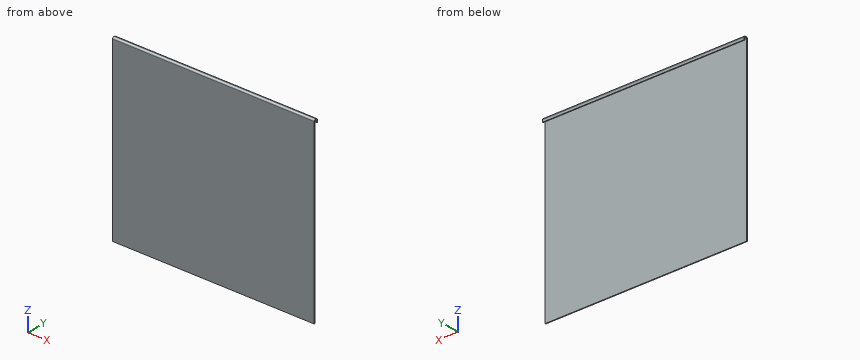
Autodesk Inventor part; units mm, degrees
ref_plane "YZ Plane" through (0, 0, 0) normal (1, 0, 0) x (0, 1, 0)
ref_plane "XZ Plane" through (0, 0, 0) normal (0, 1, 0) x (-1, 0, 0)
ref_plane "XY Plane" through (0, 0, 0) normal (0, 0, 1) x (1, 0, 0)
sketch "Sketch1" plane through (0, 0, 0) normal (0, 1, 0) x (-1, 0, 0)
  line L0 (0, 0) -> (1371.6, 0)
  line L1 (1371.6, 0) -> (1371.6, 1219.2)
  line L2 (1371.6, 1219.2) -> (0, 1219.2)
  line L3 (0, 1219.2) -> (0, 0)
  dimension "d0" = 1371.6
  dimension "d1" = 1219.2
extrude "Plate1" add sketch "Sketch1" along normal blind 5.3975
sketch "Sketch2" plane through (0, 0, 1213.8025) normal (0, 0, 1) x (1, 0, 0)
  line L0 (-1371.6, 0) -> (0, 0)
  line L1 (0, 0) -> (0, 25.4)
  line L2 (0, 25.4) -> (-1371.6, 25.4)
  line L3 (-1371.6, 25.4) -> (-1371.6, 0)
edge flange "Flange1" height 25.4 angle 90 thickness 5.3975 bend radius 5.3975 thickness toward (0, 0, 1) relief tear relief width 5.3975 relief depth 2.6987 edges at (-685.8, 5.3975, 1219.2) wall of the first edge with corners at (-1371.6, 0, 1213.8025) (0, 0, 1213.8025) (0, 25.4, 1213.8025) (-1371.6, 25.4, 1213.8025)
bend "Bend1"
corner "Corner1"
sketch "Sketch3" plane through (0, 20.0025, 1219.2) normal (0, 1, 0) x (-1, 0, 0)
  line L0 (1371.6, 0) -> (0, 0)
  line L1 (0, 0) -> (0, -25.4)
  line L2 (0, -25.4) -> (1371.6, -25.4)
  line L3 (1371.6, -25.4) -> (1371.6, 0)
edge flange "Flange2" height 25.4 angle 90 thickness 5.3975 bend radius 5.3975 thickness toward (0, 1, 0) relief tear relief width 5.3975 relief depth 2.6987 edges at (-685.8, 25.4, 1213.8025) wall of the first edge with corners at (-1371.6, 20.0025, 1219.2) (0, 20.0025, 1219.2) (0, 20.0025, 1193.8) (-1371.6, 20.0025, 1193.8)
bend "Bend2"
corner "Corner2"
equation "\"d3\" = BendReliefWidth"
equation "\"d4\" = BendReliefDepth"
equation "\"d5\" = MinimumRemnant"
equation "\"d6\" = BendRadius"
equation "\"d9\" = BendRadius"
equation "\"d10\" = CornerReliefSize"
equation "\"d11\" = GapSize"
equation "\"d12\" = JacobiRadiusSize"
equation "\"d13\" = BendReliefWidth"
equation "\"d14\" = BendReliefDepth"
equation "\"d15\" = MinimumRemnant"
equation "\"d16\" = BendRadius"
equation "\"d19\" = BendRadius"
equation "\"d20\" = CornerReliefSize"
equation "\"d21\" = GapSize"
equation "\"d22\" = JacobiRadiusSize"
equation "\"BendRadius\" = Thickness"
equation "\"BendReliefWidth\" = Thickness"
equation "\"BendReliefDepth\" = 0.5 * Thickness"
equation "\"CornerReliefSize\" = 4 * Thickness"
equation "\"MinimumRemnant\" = 2 * Thickness"
equation "\"TransitionRadius\" = BendRadius"
equation "\"JacobiRadiusSize\" = BendRadius"
equation "\"GapSize\" = Thickness"
equation "\"d2\" = BendRadius"
properties material "Polycarbonate, Clear"
Check sheet for the modelled part. Datum: model origin and axes. Units: mm. Coordinates: 2 decimals unless noted, no trailing zeros. Write each loop counter-clockwise with the first axis right and the second up, starting at its lowest first coordinate (ties: lowest second). Pieces come first, ordered by that corner, then holes. Notation, with made-up numbers: (-30.5, -8) -> (27.5, -8) arc R22 ccw to (27.5, 16) -> close; hole circle Ø8 at (-24.5, 39.25). An arc over 180 degrees is marked (long way). Use a Markdown table: item, result.
1. Sectioned sample at B-B (z = 830). Enter the section's corners in (x, y).
Reported:
| item | result |
|---|---|
| outline | (-1371.6, 0) -> (0, 0) -> (0, 5.4) -> (-1371.6, 5.4) -> close |
2. Go/stop test with flat-tipped pins: pin 1 Ø1.1 at (x, y) = (-381.5, 12) entering from -Z; pin 2 Ø1.5 at (y, z) = (8, 560) entering from -X; pin 3 Ø6 at (x, y) = (-451, 22.5) entering from -Z; pin 4 Ø4 at (x, z) = (-451.5, 549) entering from +Y. Record where each tip stops, or that it passes through.
Reported:
| item | result |
|---|---|
| pin 1 | stops at z = 1213.8 |
| pin 2 | passes through |
| pin 3 | stops at z = 1193.8 |
| pin 4 | stops at y = 5.4 |
3. Scan lines: line 1 along Z through (x, y) = (-224, 15.25); line 2 along Y through (x, z) = (-1130.5, 261); line 3 along Z through (x, y) = (-891, 18.5). Record each from-to range of solid material in increasing order.
Reported:
| item | result |
|---|---|
| line 1 | z = 1213.76 to 1219.18 |
| line 2 | y = 0 to 5.4 |
| line 3 | z = 1212.14 to 1218.47 |
4. Sectioned sample at A-A (x = -687.5). Enter the section's corners in (y, z) (1 decimal).
Reported:
| item | result |
|---|---|
| outline | (0, 0) -> (5.4, 0) -> (5.4, 1208.4) arc R5.4 cw to (10.8, 1213.8) -> (14.6, 1213.8) arc R5.4 cw to (20, 1208.4) -> (20, 1193.8) -> (25.4, 1193.8) -> (25.4, 1208.4) arc R10.8 ccw to (14.6, 1219.2) -> (10.8, 1219.2) arc R10.8 ccw to (0, 1208.4) -> close |
